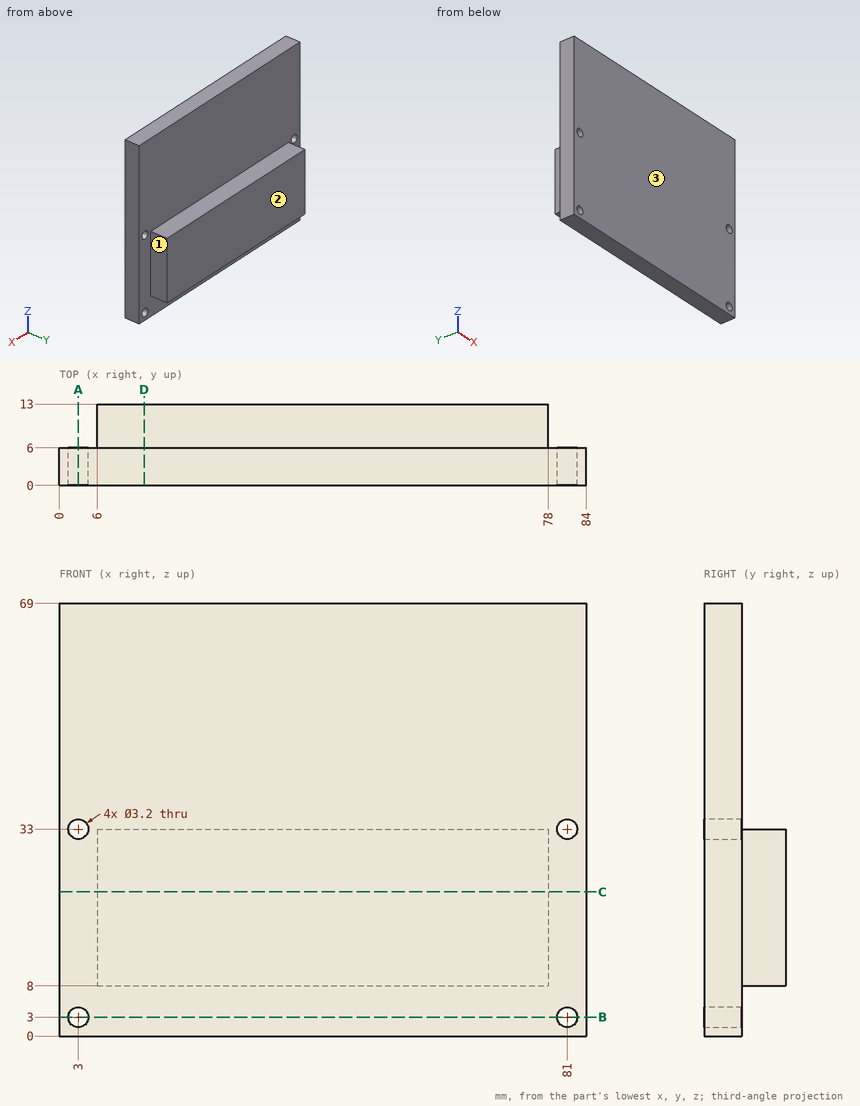
Input: dimensioned drawing with shaded views. Units: mm. Origin: part minimum x, y, z. Round coordinates to 2 decimals unless told otherwise and drop trailing zeros. Loops run counter-clockwise (first coordinate to the right, second up) from the corner with the lowest first, then second, coordinate; pieces in that order, holes last. Notation, with made-up numbers: (-33, 81) -> (-3, 81) arc R13 cw to (-3, 96) -> close; hole circle Ø9 at (36, -40). An arc over 180 degrees is marked (long way). Use one line per item in the form item = value. Start each with the question number.
1) Line query: L1, parallel to X at y = 2.75, z = 3; L2, parallel to Z at x = 81, y = 1.35; L3, parallel to Z at x = 4, y = 1. Output: solid intervals per line, ascending.
2) Section D-D on x = 13.5. Output: boundary loops of the cut face in (y, z).
3) Draft query along Y for the marked faces 1, 2 and 3. Return one class per face: released by +Y, released by -Y, zero draft, split by the parting line, or undercut.
4) Section A-A on x = 3. Output: boundary loops of the cut face in (y, z), then the cut area to 3 significant figures.
5) Section C-C on z = 23. Output: boundary loops of the cut face in (x, y).
6) First-contact query: P1, Ø2, axis at x = 55.5, y = 10.5, coming from the -Z side; P2, Ø2, axis at x = 44, y = 9.5, coming from the +Z side; P3, Ø4, axis at y = 9.5, z = 31.5, coming from the -X side. Flat tips, straight axial feed; report the tip coordinate or a pass-through.
7) Section B-B on z = 3. Output: boundary loops of the cut face in (x, y).
Response:
q1.L1 = 0 to 1.4, 4.6 to 79.4, 82.6 to 84
q1.L2 = 0 to 1.4, 4.6 to 31.4, 34.6 to 69
q1.L3 = 0 to 1.75, 4.25 to 31.75, 34.25 to 69
q2.outline = (0, 0) -> (6, 0) -> (6, 8) -> (13, 8) -> (13, 33) -> (6, 33) -> (6, 69) -> (0, 69) -> close
q3.face_1 = zero draft
q3.face_2 = released by +Y
q3.face_3 = released by -Y
q4.outline = (0, 0) -> (6, 0) -> (6, 1.4) -> (0, 1.4) -> close; (0, 4.6) -> (6, 4.6) -> (6, 31.4) -> (0, 31.4) -> close; (0, 34.6) -> (6, 34.6) -> (6, 69) -> (0, 69) -> close
q4.area = 376 mm^2
q5.outline = (0, 0) -> (84, 0) -> (84, 6) -> (78, 6) -> (78, 13) -> (6, 13) -> (6, 6) -> (0, 6) -> close
q6.P1 = 8
q6.P2 = 33
q6.P3 = 6
q7.outline = (0, 0) -> (1.4, 0) -> (1.4, 6) -> (0, 6) -> close; (4.6, 0) -> (79.4, 0) -> (79.4, 6) -> (4.6, 6) -> close; (82.6, 0) -> (84, 0) -> (84, 6) -> (82.6, 6) -> close
